```python
from build123d import *

# Parameters (mm, degrees)
SKETCH1_R           = 13.5
BOSS_EXTRUDE1_DEPTH = 30
SKETCH2_R           = 1.25
CUT_EXTRUDE1_DEPTH  = 4
SCALE1_SCALE        = 0.5


with BuildPart() as part:
    # Sketch1 → Boss-Extrude1 (new, symmetric)
    with BuildSketch(Plane(origin=(0, 0, 0), x_dir=(0, 0, -1), z_dir=(1, 0, 0))):
        Circle(SKETCH1_R)
    extrude(amount=BOSS_EXTRUDE1_DEPTH, both=True)

    # Sketch2 → Cut-Extrude1 (cut)
    with BuildSketch(Plane.ZY.offset(30)):
        with Locations((0, 10)):
            Circle(SKETCH2_R)
        with Locations((8.660254038, 5)):
            Circle(SKETCH2_R)
        with Locations((8.660254038, -5)):
            Circle(SKETCH2_R)
        with Locations((0, -10)):
            Circle(SKETCH2_R)
        with Locations((-8.660254038, -5)):
            Circle(SKETCH2_R)
        with Locations((-8.660254038, 5)):
            Circle(SKETCH2_R)
    cut_extrude1 = extrude(amount=-CUT_EXTRUDE1_DEPTH, mode=Mode.SUBTRACT)

    # Mirror1: Cut-Extrude1 across plane
    add(cut_extrude1.mirror(Plane(origin=(0, 0, 0), x_dir=(0, 0, 1), z_dir=(1, 0, 0))), mode=Mode.SUBTRACT)


with BuildPart() as part_1:
    # Scale1: scaled about (0, 0, 0)
    add(part.part.scale(SCALE1_SCALE))


solid = part_1.part
```
Here's how the part is built. I have some questions about the finished solid (model axes, mm). A direction names the side the tool comes from. Round coordinates to 2 decimals unless told otherwise and drop trailing zeros. Write each loop counter-clockwise with the first axis right and the second up, starting at its lowest first coordinate (ties: lowest second). Pieces come first, ordered by that corner, then holes. Notation, with made-up numbers: M 68,-33.5 L 79,-33.5 A30 ccw 79,4.5 Z; hole C 38,6 d5. An arc over 180 degrees is marked long. Answer as CSV lines item,"result". Start each with the question number.
1. Suppose I cut it at C-C on y = 2.5. Write out the boundary of the cut face in (x, z).
2. Thinking about a two-plate mould opening in Z: for faces 3 (the flat face through (13, 5, 0)), 4 (the flat face through (15, 0, 0)), which applies, released by +Z, released by -Z, zero draft, split by the parting line, or undercut?
3. Suppose I cut it at B-B on x = -3. Write out the boundary of the cut face in (y, z).
4. On a 3-axis mill with a long thin cutter (end or side, diameter ignored), from which of +Z, -Z, +X, -X, +Y, -Y can I reach the whole of each face in a straight line? I mean faces 1 (the cylindrical face through (14.014, -4.473, 0.336)), 2 (the flat face through (-13, -2.5, 4.3)). Say none if no direction works.
5. I need wall thicknesses on probe 1 along Y at (x, z) = (-14.15, 0) (3 decimals); probe 2 along Y at (x, z) = (-10, 0.25). Which ranges of each line are inside material? Lowest first, please.
6. Suppose I cut it at A-A on z = 0. Write out the boundary of the cut face in (x, y) (3 decimals).
7. Suppose I cut it at D-D on y = 5. Write out the boundary of the cut face in (x, z) (3 decimals), then the cut area to 3 significant figures.
8. I'm going to push flat-ended pins straight in: pin 1 Ø0.8 at (y, z) = (2.5, 4.33) entering from -X; pin 2 Ø4 at (x, y) = (-1.5, -2.5) entering from -Z; pin 3 Ø0.6 at (y, z) = (-5, 0) entering from +X. Where does each tip first touch, or does it pass through?
Check result:
1,outline,"M -15,-6.27 L 15,-6.27 L 15,-4.96 L 13,-4.96 L 13,-3.71 L 15,-3.71 L 15,3.71 L 13,3.71 L 13,4.96 L 15,4.96 L 15,6.27 L -15,6.27 L -15,4.96 L -13,4.96 L -13,3.71 L -15,3.71 L -15,-3.71 L -13,-3.71 L -13,-4.96 L -15,-4.96 Z"
2,face 3,"undercut"
2,face 4,"zero draft"
3,outline,"C 0,0 d13.5"
4,face 1,"+X"
4,face 2,"-X"
5,probe 1,"y = -6.75 to -5.625, -4.375 to 4.375, 5.625 to 6.75"
5,probe 2,"y = -6.75 to 6.75"
6,outline,"M -15,-6.75 L 15,-6.75 L 15,-5.625 L 13,-5.625 L 13,-4.375 L 15,-4.375 L 15,4.375 L 13,4.375 L 13,5.625 L 15,5.625 L 15,6.75 L -15,6.75 L -15,5.625 L -13,5.625 L -13,4.375 L -15,4.375 L -15,-4.375 L -13,-4.375 L -13,-5.625 L -15,-5.625 Z"
7,outline,"M -15,-4.535 L 15,-4.535 L 15,-0.625 L 13,-0.625 L 13,0.625 L 15,0.625 L 15,4.535 L -15,4.535 L -15,0.625 L -13,0.625 L -13,-0.625 L -15,-0.625 Z"
7,area,"267 mm2"
8,pin 1,"stops at x = -13"
8,pin 2,"stops at z = -6.73"
8,pin 3,"stops at x = 13"
